Geometry: see drawing. Coordinates: mm, zero at the bounding-box minimum. A direction names the side the tool comes from. Give positions to 0.01 mm unless a question says otherwise; leave off trailing zeros. Write each loop counter-clockwise with the first axis right and the second up, starting at its lowest first coordinate (ties: lowest second). Pieces come first, ordered by that corner, then holes. Notation, with made-up numbers: (44, 15) -> (97, 15) arc R16 ccw to (97, 35) -> close; hole circle Ø9 at (7, 68). An arc over 180 degrees is marked (long way). Use one line per item in the form item = value. Start each with the question number.
(1) Draft query along X for the marked faces 4, 5 and 6. Return one class per face: pulls with the +X half, pulls with the -X half, needs draft (parallel to the pull), parting line crosses it, or undercut.
(2) Set-up query: the marked faces 1, 2 and 3. Return all of +Z, -Z, +X, -X, +Y, -Y with unobstructed straight access to the full face (end or side cutting, diameter ignored); none if empty.
(3) Cut plane A-A, the plane x = 19. Output: boundary loops of the cut face in (y, z).
(4) Cut plane B-B, the plane z = 19. Output: boundary loops of the cut face in (x, y), and give its area (3 significant figures).
(5) Material intervals for line 1 along X through (y, z) = (33.5, 20.95) (3 decimals); line 2 along Y through (x, z) = (19, 9.5); line 3 along Y through (x, z) = (19, 20.3), sorted ascending. Write a range as from..to.
(6) First-contact query: P1, Ø3.5, axis at x = 33.5, y = 4.5, coming from the +Z side; P2, Ø8.5, axis at x = 4.5, y = 33.5, coming from the -Z side; P3, Ø4.5, axis at x = 33.5, y = 33.5, coming from the +Z side; P4, Ø3, axis at x = 12, z = 3.5, coming from the -Y side. Flat tips, straight axial feed; report the tip coordinate or a pass-through.
(7) Cut plane D-D, the plane y = 34.5. Output: boundary loops of the cut face in (x, z), and give its area (3 significant figures).
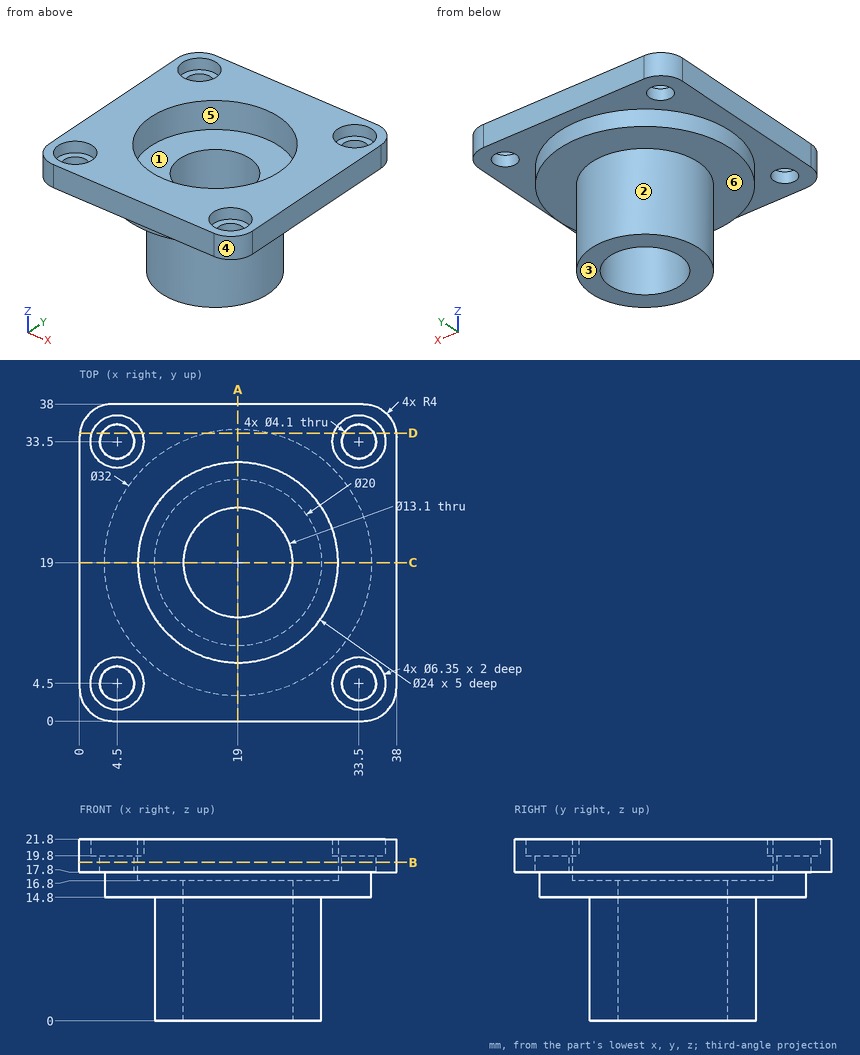
Geometry says:
q1.face_4 = pulls with the +X half
q1.face_5 = undercut
q1.face_6 = needs draft
q2.face_1 = +Z
q2.face_2 = -Z
q2.face_3 = -Z, +X, -X, +Y, -Y
q3.outline = (0, 17.8) -> (3, 17.8) -> (3, 14.8) -> (9, 14.8) -> (9, 0) -> (12.45, 0) -> (12.45, 16.8) -> (7, 16.8) -> (7, 21.8) -> (0, 21.8) -> close; (25.55, 0) -> (29, 0) -> (29, 14.8) -> (35, 14.8) -> (35, 17.8) -> (38, 17.8) -> (38, 21.8) -> (31, 21.8) -> (31, 16.8) -> (25.55, 16.8) -> close
q4.outline = (0, 4) arc R4 ccw to (4, 0) -> (34, 0) arc R4 ccw to (38, 4) -> (38, 34) arc R4 ccw to (34, 38) -> (4, 38) arc R4 ccw to (0, 34) -> close; hole circle Ø4.1 at (4.5, 4.5); hole circle Ø4.1 at (4.5, 33.5); hole circle Ø24 at (19, 19); hole circle Ø4.1 at (33.5, 4.5); hole circle Ø4.1 at (33.5, 33.5)
q4.area = 925 mm^2
q5.line_1 = 0..1.325, 7.675..30.325, 36.675..38
q5.line_2 = 9..12.45, 25.55..29
q5.line_3 = 0..7, 31..38
q6.P1 = through
q6.P2 = 17.8
q6.P3 = 19.8
q6.P4 = 10.65
q7.outline = (0.03, 17.8) -> (2.71, 17.8) -> (2.71, 19.8) -> (1.49, 19.8) -> (1.49, 21.8) -> (0.03, 21.8) -> close; (6.29, 17.8) -> (15.03, 17.8) -> (15.03, 14.8) -> (22.97, 14.8) -> (22.97, 17.8) -> (31.71, 17.8) -> (31.71, 19.8) -> (30.49, 19.8) -> (30.49, 21.8) -> (7.51, 21.8) -> (7.51, 19.8) -> (6.29, 19.8) -> close; (35.29, 17.8) -> (37.97, 17.8) -> (37.97, 21.8) -> (36.51, 21.8) -> (36.51, 19.8) -> (35.29, 19.8) -> close
q7.area = 137 mm^2
